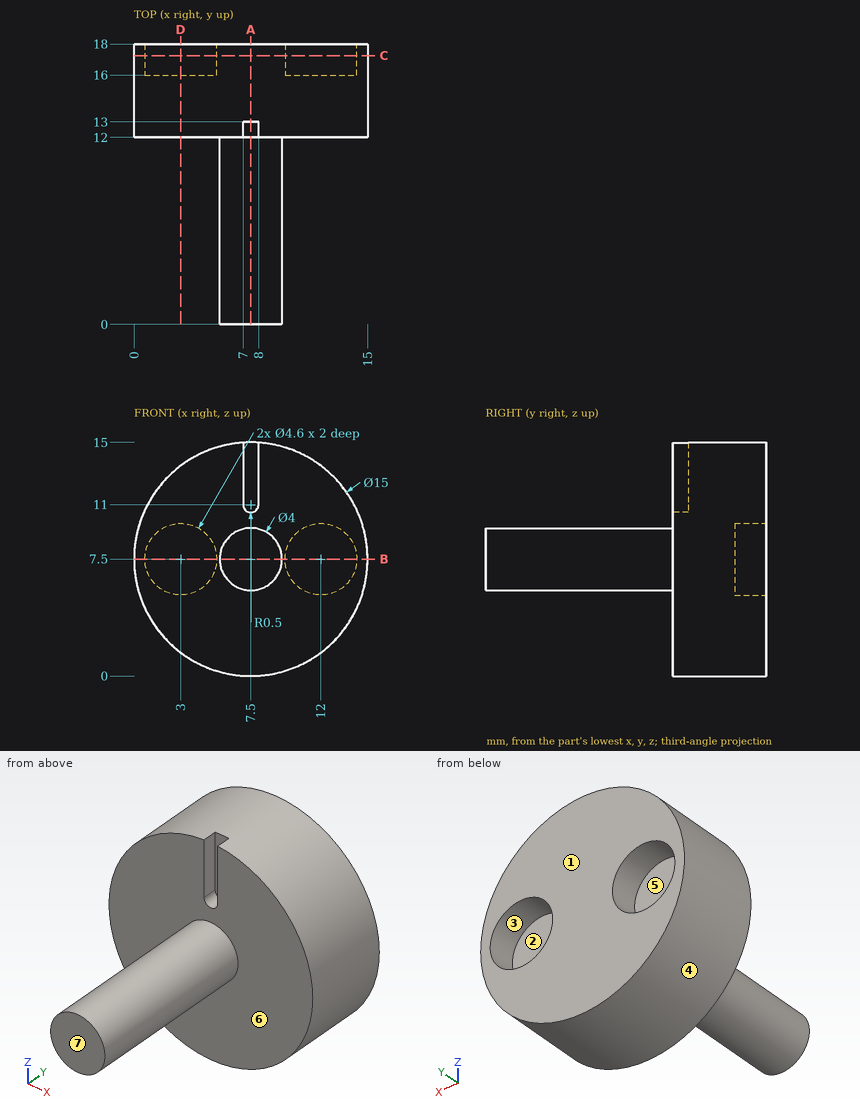
Answer from the drawing. Dimensions are ordinates in mm from the lowest x, y and z of the part. A direction names the side the tool comes from. Coordinates: 2 decimals unless noted, no trailing zeros. Write each loop counter-clockwise with the first axis right and the second up, starting at its lowest first coordinate (ties: lowest second). Pieces come first, ordered by that corner, then holes. Notation, with made-up numbers: (10, 85) - (44, 85) arc R19 ccw to (44, 99) - close; hole circle Ø2 at (1, 61.5). An arc over 180 degrees is marked (long way). Return JSON: item names as keys, results as strings. Group by question number.
Q1. The part is cut by section A-A on x = 7.5. Write down the section's boundary in (y, z).
Q2. Find the intervals of material crossed by line 1 along Y through (x, z) = (5.5, 6); line 2 along Z through (x, y) = (3, 17.1); line 3 along Y through (x, z) = (12.25, 7.75), in increasing order. Write a range as [from, to].
Q3. The part is cut by section C-C on y = 17.25. Write down the section's boundary in (x, z).
Q4. The part is cut by section B-B on z = 7.5. Write down the section's boundary in (x, y), and give its area (3 significant figures).
Q5. For a pull along X with two mould halves and no side action, classify the marked faces 1, 2, 3 and 4 as +X half, -X half, draft (parallel to the pull), parting line (faces both ways), or undercut.
Q6. Which of the six approach directions +Z, -Z, +X, -X, +Y, -Y give full straight-line access (tool end or side, diameter ignored) to the marked faces 5, 6 and 7?
Q7. Flat-ended cylindrical pins translate along their axes: pin 1 Ø5 at (y, z) = (8.5, 9) entering from +X; pin 2 Ø6 at (y, z) = (7.5, 5) entering from -X; pin 3 Ø6 at (y, z) = (9.5, 13.5) entering from -X. Find the tip coordinate at first contact, or state that the pin passes through.
Q8. The part is cut by section D-D on x = 3. Write down the section's boundary in (y, z), and give its area (3 significant figures).
Evaluation:
{
 "1": {"outline": "(0, 5.5) - (12, 5.5) - (12, 0) - (18, 0) - (18, 15) - (13, 15) - (13, 10.5) - (12, 10.5) - (12, 9.5) - (0, 9.5) - close"},
 "2": {"line 1": "y = [12, 18]", "line 2": "z = [1.5, 5.2], [9.8, 13.5]", "line 3": "y = [12, 16]"},
 "3": {"outline": "circle Ø15 at (7.5, 7.5); hole circle Ø4.6 at (3, 7.5); hole circle Ø4.6 at (12, 7.5)"},
 "4": {"outline": "(0, 12) - (5.5, 12) - (5.5, 0) - (9.5, 0) - (9.5, 12) - (15, 12) - (15, 18) - (14.3, 18) - (14.3, 16) - (9.7, 16) - (9.7, 18) - (5.3, 18) - (5.3, 16) - (0.7, 16) - (0.7, 18) - (0, 18) - close", "area": "120 mm2"},
 "5": {"face 1": "draft", "face 2": "undercut", "face 3": "undercut", "face 4": "parting line"},
 "6": {"face 5": "+Y", "face 6": "-Y", "face 7": "+Z, -Z, +X, -X, -Y"},
 "7": {"pin 1": "stops at x = 9.5", "pin 2": "stops at x = 5.5", "pin 3": "stops at x = 1.38"},
 "8": {"outline": "(12, 1.5) - (18, 1.5) - (18, 5.2) - (16, 5.2) - (16, 9.8) - (18, 9.8) - (18, 13.5) - (12, 13.5) - close", "area": "62.8 mm2"}
}
